Can you work these out from the model? Positions are in its coordinate system, mm. A direction names the side the tool comes from. Give positions to 0.01 mm unless a question says otherwise; leave off trailing zeros. Loops run counter-clockwise (first coordinate to the right, second up) from the corner with the lowest first, then second, coordinate; pieces in that order, holes last. Notation, with made-up numbers: (11.25, -18.75) -> (54.25, -18.75) arc R15 cw to (54.25, -11.75) -> close; hole circle Ø11 at (-15, 87). An arc over 180 degrees is marked (long way). Return JSON: item names as keys, results as strings. Group by question number.
Q1. Suppose I cut it at A-A, the plane y = 16. Please give me the cut outline in (x, z), and give its area (3 significant figures).
Q2. Thinking about a two-plate mould opening in X: for faces 1 (the flat face through (-7.044, 61.495, -21.475)), 2 (the flat face through (21.72, 62.44, 3.49)), 3 (the flat face through (-2, 63, 22.5)), which applies, pulls with the +X half, pulls with the -X half, needs draft (parallel to the pull), parting line crosses it, or undercut?
Q3. Which directions (+Z, -Z, +X, -X, +Y, -Y) give clear straight access to the entire face, cutting with the end or side of a thin tool? Please do faces 4 (the flat face through (18.321, 61.495, 13.234)), 5 (the flat face through (-6.924, 61, 22)), 6 (the cylindrical face through (-13.18, 62.34, 14.37)).
Q4. Will these pins go through, and if not, where does the flat tip stop? pin 1 (1.5 mm diameter, centred on x = -2.5, z = -14, fed in from +Y); pin 2 (10 mm diameter, centred on x = 14.5, y = 62.5, fed in from +Z); pin 3 (3 mm diameter, centred on y = 62, z = -9.5, fed in from +X); pin 4 (21.5 mm diameter, centred on x = -6.5, z = 10.5, fed in from -Y).
Q5. I need wall thicknesses on line 1 along X through (y, z) = (2.2, 0); line 2 along Y through (x, z) = (-16, -3.5); line 3 along X through (y, z) = (0.6, 0). Which ranges of each line are inside material? Lowest first, please. Write a range as [from, to].
```python
from build123d import *

# Parameters (mm, degrees)
SHELL5_T            = -2
FILLET1_R           = 10
BOSS_EXTRUDE1_DEPTH = 1
CIRPATTERN1_COUNT   = 5


with BuildPart() as part:
    # Sketch1 → Revolve1 (revolve)
    with BuildSketch(Plane.XY, mode=Mode.PRIVATE) as revolve1_sk:
        Polygon((20, 0), (20, 58.690524981), (21.5, 58.690524981), (21.5, 64.190524981), (20, 70), (0, 70), (0, 2.938550041), (5, 2.938550041), (5, 1.5), (19, 1.5), (19, 0), align=None)
    revolve(revolve1_sk.sketch.rotate(Axis((0, 0, 0), (0, 1, 0)), 90), axis=Axis((0, 0, 0), (0, 1, 0)))

    # Shell5
    shell5_openings = [part.faces().sort_by_distance(p)[0] for p in [
        (0, 70, 0),
    ]]
    offset(amount=SHELL5_T, openings=shell5_openings, kind=Kind.INTERSECTION)

    # Fillet1
    # the kernel refuses this fillet: 10 mm, written as the material it takes off along each edge
    with BuildSketch(Plane(origin=(0, 60.690524981, 0), x_dir=(0, 0, -1), z_dir=(1, 0, 0))) as fillet1_piece_1:
        with BuildLine():
            CenterArc((28, -5.267826876), FILLET1_R, 148.211669383, 31.788330617)
            Line((19.5, 0), (19.33, 0.105356538))
            ThreePointArc((19.33, 0.105356538), (18.75, 0.2), (18, 0.2))
            Line((18, 0.2), (17.8, 0))
            Line((17.8, 0), (17.8, -5.267826876))
            Line((17.8, -5.267826876), (18, -5.267826876))
        make_face()
    revolve(axis=Axis((0, 60.690524981, 0), (0, 1, 0)), mode=Mode.SUBTRACT)

    # Sketch4 → Boss-Extrude1 (add, symmetric)
    with BuildSketch(Plane.XY.offset(21.5)):
        Polygon((-2.224405673, 61.290524981), (7.075594327, 63.190524981), (7.075594327, 64.190524981), (-6.924405673, 64.190524981), (-6.924405673, 58.723404538), (-5.724405673, 58.690524981), (-5.724405673, 62.790524981), (-2.224405673, 62.790524981), align=None)
    boss_extrude1 = extrude(amount=BOSS_EXTRUDE1_DEPTH, both=True)

    # CirPattern1: Boss-Extrude1 ×5 about axis
    cirpattern1_axis = Axis((0, 0, 0), (0, 1, 0))
    for i in range(1, CIRPATTERN1_COUNT):
        add(boss_extrude1.rotate(cirpattern1_axis, i * 360 / CIRPATTERN1_COUNT))


solid = part.part
```
Ans:
{
 "1": {"outline": "circle Ø40 at (0, 0); hole circle Ø36 at (0, 0)", "area": "239 mm^2"},
 "2": {"face 1": "undercut", "face 2": "pulls with the +X half", "face 3": "needs draft"},
 "3": {"face 4": "+Z, +Y, -Y", "face 5": "+Z, -X, +Y, -Y", "face 6": "none"},
 "4": {"pin 1": "stops at y = 3.5", "pin 2": "stops at z = 19.29", "pin 3": "stops at x = 19.96", "pin 4": "stops at y = 0"},
 "5": {"line 1": "x = [-20, -5], [5, 20]", "line 2": "y = [1.5, 3.5]", "line 3": "x = [-20, -19], [19, 20]"}
}
